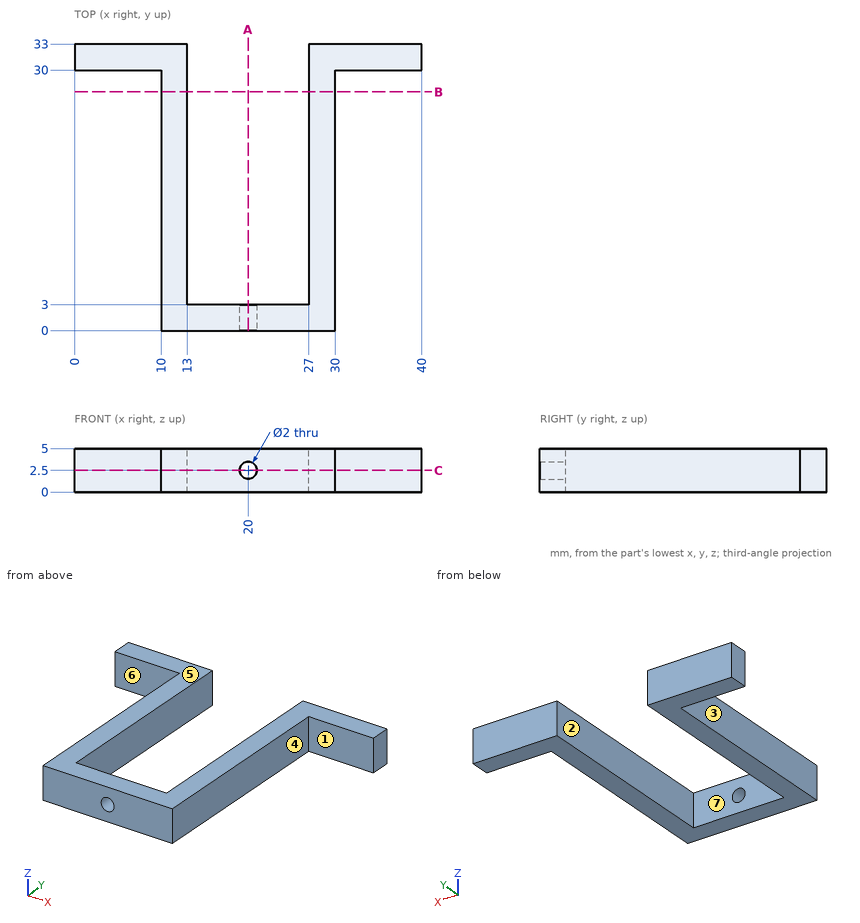
Could you check a few things on this drawing? It's one solid part, dimensions in mm from its lowest x, y, z. A direction names the side the tool comes from. Give positions to 0.01 mm unless a question says otherwise; leave off trailing zeros. Order: outer loops, then holes, each group sorted by start corner. A loop starts at its lowest first (then second) coordinate and runs counter-clockwise, first axis right, second up.
1. Suppose I cut it at A-A (x = 20). Write out the boundary of the cut face in (y, z), plus the area to 3 significant figures.
Answers below:
outline: (0, 0) - (3, 0) - (3, 1.5) - (0, 1.5) - close; (0, 3.5) - (3, 3.5) - (3, 5) - (0, 5) - close
area: 9.00 mm2
2. Which directions (+Z, -Z, +X, -X, +Y, -Y) give clear straight access to the entire face, cutting with the end or side of a thin tool? Please do the marked faces 5, 6 and 7.
Answers below:
face 5: +Z, +X, -X, +Y, -Y
face 6: +Z, -Z, -X, -Y
face 7: +Z, -Z, +Y
3. Suppose I cut it at B-B (y = 27.5). Write out the boundary of the cut face in (x, z), plus the area to 3 significant figures.
Answers below:
outline: (10, 0) - (13, 0) - (13, 5) - (10, 5) - close; (27, 0) - (30, 0) - (30, 5) - (27, 5) - close
area: 30.0 mm2
4. For pin 1 (3 mm diameter, centred on y = 16, z = 2.5, fed in from -X); pin 2 (2.5 mm diameter, centred on y = 22.5, z = 2.5, fed in from +X); pin 3 (4 mm diameter, centred on x = 23, y = 6, fed in from +Z); pin 4 (2 mm diameter, centred on x = 30.5, y = 10.5, fed in from +Z), each with a flat end and sliding along its axis, tell me the tip position at first contact or that it passes through.
Answers below:
pin 1: stops at x = 10
pin 2: stops at x = 30
pin 3: passes through
pin 4: stops at z = 5
5. Suppose I cut it at C-C (z = 2.5). Write out the boundary of the cut face in (x, y).
Answers below:
outline: (0, 30) - (10, 30) - (10, 0) - (19, 0) - (19, 3) - (13, 3) - (13, 33) - (0, 33) - close; (21, 0) - (30, 0) - (30, 30) - (40, 30) - (40, 33) - (27, 33) - (27, 3) - (21, 3) - close
6. I need wall thicknesses on L1, parallel to X at y = 25.5, z = 0.95; L2, parallel to X at y = 0.65, z = 2.5; L3, parallel to Z at x = 20, y = 0.6. Which ranges of each line are inside material? Lowest first, please.
Answers below:
L1: x = 10 to 13, 27 to 30
L2: x = 10 to 19, 21 to 30
L3: z = 0 to 1.5, 3.5 to 5
7. Thinking about a two-plate mould opening in X: for the marked faces 1, 2, 3 and 4, which applies, +X half, -X half, draft (parallel to the pull), parting line (faces both ways), or undercut?
Answers below:
face 1: draft
face 2: undercut
face 3: -X half
face 4: +X half
